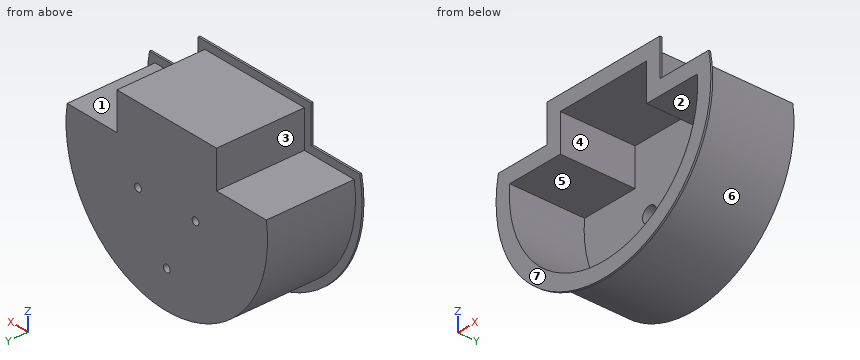
```python
from build123d import *

# Parameters (mm, degrees)
EXTRUIR_L_MINA1_DEPTH   = 20
SALIENTE_EXTRUIR1_DEPTH = 4
CROQUIS3_R              = 2.1
CORTAR_EXTRUIR2_DEPTH   = 2.2
SALIENTE_EXTRUIR3_DEPTH = 0.5
CROQUIS5_R              = 1
CORTAR_EXTRUIR3_DEPTH   = 10


with BuildPart() as part:
    # Croquis1 → Extruir-Lámina1 (new body)
    with BuildSketch(Plane(origin=(0, 0, 0), x_dir=(1, 0, 0), z_dir=(0, 1, 0))):
        with BuildLine():
            Line((-30, 10), (-15, 10))
            Line((-15, 10), (-15, 0))
            Line((-15, 0), (15, 0))
            Line((15, 0), (15, 10))
            Line((15, 10), (30, 10))
            ThreePointArc((30, 10), (0, 45), (-30, 10))
        make_face()
        with BuildLine():
            Line((-28.233718443, 12), (-13, 12))
            Line((-13, 12), (-13, 2))
            Line((-13, 2), (13, 2))
            Line((13, 2), (13, 12))
            Line((13, 12), (28.233718443, 12))
            ThreePointArc((28.233718443, 12), (0, 43), (-28.233718443, 12))
        make_face(mode=Mode.SUBTRACT)
    extrude(amount=EXTRUIR_L_MINA1_DEPTH)

    # Croquis2 → Saliente-Extruir1 (add)
    with BuildSketch(Plane(origin=(0, 20, 0), x_dir=(1, 0, 0), z_dir=(0, 1, 0))):
        with BuildLine():
            Line((15, 10), (30, 10))
            ThreePointArc((30, 10), (0, 45), (-30, 10))
            Line((-30, 10), (-15, 10))
            Line((-15, 10), (-15, 0))
            Line((-15, 0), (15, 0))
            Line((15, 0), (15, 10))
        make_face()
    extrude(amount=SALIENTE_EXTRUIR1_DEPTH)

    # Croquis3 → Cortar-Extruir2 (cut)
    with BuildSketch(Plane.XZ.offset(-20)):
        with Locations(Location((-8.660254038, -20, 0), (0, 0, 270))):
            Circle(CROQUIS3_R)
        with Locations(Location((8.660254038, -20, 0), (0, 0, 270))):
            Circle(CROQUIS3_R)
        with Locations(Location((0, -35, 0), (0, 0, 270))):
            Circle(CROQUIS3_R)
    extrude(amount=-CORTAR_EXTRUIR2_DEPTH, mode=Mode.SUBTRACT)

    # Croquis4 → Saliente-Extruir3 (add)
    with BuildSketch(Plane.XZ):
        with BuildLine():
            Line((17, 2), (-17, 2))
            Line((-17, 2), (-17, -8))
            Line((-17, -8), (-31.667919775, -8))
            ThreePointArc((-31.667919775, -8), (0, -47), (31.667919775, -8))
            Line((31.667919775, -8), (17, -8))
            Line((17, -8), (17, 2))
        make_face()
        with BuildLine():
            Line((13, -12), (28.233718443, -12))
            ThreePointArc((28.233718443, -12), (0, -43), (-28.233718443, -12))
            Line((-28.233718443, -12), (-13, -12))
            Line((-13, -12), (-13, -2))
            Line((-13, -2), (13, -2))
            Line((13, -2), (13, -12))
        make_face(mode=Mode.SUBTRACT)
    extrude(amount=-SALIENTE_EXTRUIR3_DEPTH)

    # Croquis5 → Cortar-Extruir3 (cut)
    with BuildSketch(Plane.XZ.offset(-20)):
        with Locations(Location((-8.660254038, -20, 0), (0, 0, 270))):
            Circle(CROQUIS5_R)
        with Locations(Location((8.660254038, -20, 0), (0, 0, 270))):
            Circle(CROQUIS5_R)
        with Locations(Location((0, -35, 0), (0, 0, 270))):
            Circle(CROQUIS5_R)
    extrude(amount=-CORTAR_EXTRUIR3_DEPTH, mode=Mode.SUBTRACT)


solid = part.part
```
Can you work these out from the model? Positions are in its coordinate system, mm. Face numbers are marked on the shaded views. A direction names the side the tool comes from. Coordinates: 2 decimals unless noted, no trailing zeros. Order: outer loops, then holes, each group sorted by start corner. A loop starts at its lowest first (then second) coordinate and runs counter-clockwise, first axis right, second up. Notation, with made-up numbers: (59.5, 51) - (104.5, 51) arc R25 ccw to (104.5, 83) - close; hole circle Ø10 at (-18.75, -37.5). An arc over 180 degrees is marked (long way). Answer in a Markdown table with one row per item.
1. For pin 1 (8 mm diameter, centred on y = 10, z = -5.5, fed in from +X); pin 2 (6 mm diameter, centred on y = 11, z = -25.5, fed in from -X); pin 3 (4.5 mm diameter, centred on x = -18, y = 9, fed in from -Z); pin 4 (3 mm diameter, centred on x = -8.66, z = -20, fed in from +Y), each with a flat end and sliding along its axis, tell me the tip position at first contact or that it passes through.
Reply:
| item | result |
|---|---|
| pin 1 | stops at x = 15 |
| pin 2 | stops at x = -29.32 |
| pin 3 | stops at z = -40.59 |
| pin 4 | stops at y = 24 |
2. Suppose I cut it at C-C (z = -35). Please give me the cut outline in (x, y).
Reply:
| item | result |
|---|---|
| outline | (-25.15, 0) - (-19.74, 0) - (-19.74, 20) - (-2.1, 20) - (-2.1, 22.2) - (-1, 22.2) - (-1, 24) - (-22.52, 24) - (-22.52, 0.5) - (-25.15, 0.5) - close; (1, 22.2) - (2.1, 22.2) - (2.1, 20) - (19.74, 20) - (19.74, 0) - (25.15, 0) - (25.15, 0.5) - (22.52, 0.5) - (22.52, 24) - (1, 24) - close |
3. Suppose I cut it at D-D (z = -20). Please give me the cut outline in (x, y), and give its area (3 significant figures).
Reply:
| item | result |
|---|---|
| outline | (-31.91, 0) - (-27.85, 0) - (-27.85, 20) - (-10.76, 20) - (-10.76, 22.2) - (-9.66, 22.2) - (-9.66, 24) - (-29.88, 24) - (-29.88, 0.5) - (-31.91, 0.5) - close; (-7.66, 22.2) - (-6.56, 22.2) - (-6.56, 20) - (6.56, 20) - (6.56, 22.2) - (7.66, 22.2) - (7.66, 24) - (-7.66, 24) - close; (9.66, 22.2) - (10.76, 22.2) - (10.76, 20) - (27.85, 20) - (27.85, 0) - (31.91, 0) - (31.91, 0.5) - (29.88, 0.5) - (29.88, 24) - (9.66, 24) - close |
| area | 297 mm^2 |
4. Suppose I cut it at B-B (y = 13.75). Please give me the cut outline in (x, z).
Reply:
| item | result |
|---|---|
| outline | (-30, -10) arc R30.36 ccw (long way) to (30, -10) - (15, -10) - (15, 0) - (-15, 0) - (-15, -10) - close; hole (-28.23, -12) arc R28.36 ccw (long way) to (28.23, -12) - (13, -12) - (13, -2) - (-13, -2) - (-13, -12) - close |
5. For the marked faces 1, 2 and 3, which set-ups out of +Z, -Z, +X, -X, +Y, -Y let a thin tool reach every point of the face, with its end or its side?
Reply:
| item | result |
|---|---|
| face 1 | +Z, +X, +Y |
| face 2 | -Y |
| face 3 | +Z, -X, +Y |
6. Suppose I cut it at A-A (x = 0). Please give me the cut outline in (y, z), and give its area (3 significant figures).
Reply:
| item | result |
|---|---|
| outline | (0, -47) - (0.5, -47) - (0.5, -45) - (24, -45) - (24, -36) - (22.2, -36) - (22.2, -37.1) - (20, -37.1) - (20, -43) - (0, -43) - close; (0, -2) - (20, -2) - (20, -32.9) - (22.2, -32.9) - (22.2, -34) - (24, -34) - (24, 0) - (0.5, 0) - (0.5, 2) - (0, 2) - close |
| area | 249 mm^2 |
7. If we mould it in two halves opening along X, with no side actions, what happens to the marked faces 4, 5, 6 and 7? For each: pulls with the +X half, pulls with the -X half, needs draft (parallel to the pull), parting line crosses it, or undercut.
Reply:
| item | result |
|---|---|
| face 4 | undercut |
| face 5 | undercut |
| face 6 | parting line crosses it |
| face 7 | needs draft |
8. If I drill on line 1 along Z through (x, y) = (0, 11.5); line 2 along X through (y, z) = (20.9, -20); line 3 along X through (y, z) = (23.4, -20), over which ranges is the centre line in solid material (lowest first)?
Reply:
| item | result |
|---|---|
| line 1 | z = -45 to -43, -2 to 0 |
| line 2 | x = -29.88 to -10.76, -6.56 to 6.56, 10.76 to 29.88 |
| line 3 | x = -29.88 to -9.66, -7.66 to 7.66, 9.66 to 29.88 |
